Solid Edge part; units mm, degrees
sketch "Sketch1" plane through (0, 0, 0) normal (0, -1, 0) x (1, 0, 0)
  circle A0 centre (80.5127, 55.3877) radius 22.5
extrude "Protrusion1" add sketch "Sketch1" against normal blind 10
sketch "Sketch2" plane through (80.5127, 10, 55.3877) normal (0, 1, 0) x (0, 0, -1)
  circle A0 centre (0, 0) radius 2.95
extrude "ExtrudedCutout_5" cut sketch "Sketch2" against normal blind 4
sketch "Sketch3" plane through (80.5127, 6, 55.3877) normal (0, 1, 0) x (-1, 0, 0)
  circle A0 centre (0, 0) radius 1.05
extrude "Cutout1" cut sketch "Sketch3" against normal up to next
sketch "Sketch4" plane through (80.5127, 5, 51.1598) normal (0, -1, 0) x (1, 0, 0)
  circle A0 centre (0, 4.2279) radius 3.55
extrude "ExtrudedCutout_7" cut sketch "Sketch4" against normal blind 0.5
chamfer "Chamfer_2" distance 1.9 distance2 0.5 1 edges at (80.5127, 6, 58.3377) measured on face at (78.605, 6, 53.362)
sketch "Sketch5" plane through (80.5127, 10, 55.3877) normal (0, 1, 0) x (0, 0, 1)
  circle A0 centre (0, 0) radius 22.5
  circle A1 centre (0, 0) radius 3
extrude "ExtrudedProtrusion_4" add sketch "Sketch5" along normal blind 1.5
sketch "Sketch6" plane through (80.5127, 0, 55.3877) normal (0, -1, 0) x (0, 0, 1)
  line L0 (1.5, 9.61) -> (1.5, 5.61)
  arc A0 (5.61, 1.5) -> (1.5, 5.61) centre (1.5, 1.5) ccw
  line L1 (5.61, 1.5) -> (9.61, 1.5)
  arc A1 (9.61, 1.5) -> (9.61, -1.5) centre (9.61, 0) cw
  line L2 (9.61, -1.5) -> (5.61, -1.5)
  arc A2 (1.4978, -5.61) -> (5.61, -1.5) centre (1.4978, -1.4978) ccw
  line L3 (1.4978, -12.31) -> (1.4978, -5.61)
  arc A3 (-1.5, -12.31) -> (1.4978, -12.31) centre (-0.0011, -13.6341) ccw
  line L4 (-1.5, -5.61) -> (-1.5, -12.31)
  arc A4 (-5.61, -1.5) -> (-1.5, -5.61) centre (-1.5, -1.5) ccw
  line L5 (-9.61, -1.5) -> (-5.61, -1.5)
  arc A5 (-9.61, 1.5) -> (-9.61, -1.5) centre (-9.61, 0) ccw
  line L6 (-5.61, 1.5) -> (-9.61, 1.5)
  arc A6 (-5.61, 1.5) -> (-1.5, 5.61) centre (-1.5, 1.5) cw
  line L7 (-1.5, 9.61) -> (-1.5, 5.61)
  arc A7 (1.5, 9.61) -> (-1.5, 9.61) centre (0, 9.61) ccw
  dimension "D1" = 1.5
  dimension "D2" = 1.5
  dimension "D3" = 5.61
  dimension "D4" = 9.61
  dimension "D5" = 5.61
  dimension "D6" = 1.5
  dimension "D7" = 1.4978
  dimension "D8" = 9.61
extrude "ExtrudedCutout_9" cut sketch "Sketch6" against normal blind 6.7
sketch "Sketch7" plane through (80.5127, 11.5, 55.3877) normal (0, 1, 0) x (0, 0, -1)
  arc A0 (-7.5, 4.5) -> (-4.5, 7.5) centre (-7.9685, 7.9685) ccw
  line L0 (-3.5, 17.5) -> (-4.5, 7.5)
  arc A1 (-3.5, 17.5) -> (3.5, 17.5) centre (0, 17.15) cw
  line L1 (3.5, 17.5) -> (4.5, 7)
  arc A2 (4.5, 7) -> (7.5, 4.5) centre (7.8596, 7.9815) ccw
  line L2 (7.5, 4.5) -> (17.5, 3.5)
  arc A3 (17.5, 3.5) -> (17.5, -3.5) centre (17.15, 0) cw
  line L3 (7.5, -4.5) -> (17.5, -3.5)
  arc A4 (4.5, -7.5) -> (7.5, -4.5) centre (7.9657, -7.9657) cw
  line L4 (4.5, -7.5) -> (3.5, -17.5)
  arc A5 (-3.5, -17.5) -> (3.5, -17.5) centre (0, -17.15) ccw
  line L5 (-4.5, -7.5) -> (-3.5, -17.5)
  arc A6 (-7.5, -4.5) -> (-4.5, -7.5) centre (-7.9685, -7.9685) cw
  line L6 (-17.5, -3.5) -> (-7.5, -4.5)
  arc A7 (-17.5, 3.5) -> (-17.5, -3.5) centre (-17.15, 0) ccw
  line L7 (-7.5, 4.5) -> (-17.5, 3.5)
extrude "ExtrudedCutout_10" cut sketch "Sketch7" against normal blind 3.5
Input: part model. Units: mm. Frame: model coordinates. A direction names the side the tool comes from. Coordinates: 2 decimals unless noted, no trailing zeros. Loops run counter-clockwise (first coordinate to the right, second up) from the corner with the lowest first, then second, coordinate; pieces in that order, holes last. Notation, with made-up numbers: M 14,52 L 46,52 A16 ccw 46,59 Z; hole C 54.5,33 d11. An arc over 180 degrees is marked long. Use a Markdown table: item, result. Add a question column.
1) Section C-C, the plane x = 65.5. Return the cut outline in (y, z).
2) Set-up query: faces 1 (the cylindrical face through (101.18, 9.77, 55.46)), 2 (the cylindrical face through (84.887, 3.303, 50.95)), 3 (the flat face through (75.8, 0, 50.7)). Return all of +Z, -Z, +X, -X, +Y, -Y with unobstructed straight access to the full face (end or side cutting, diameter ignored); none if empty.
3) Pin query (flat end, axial travel): P1, Ø4.5, axis at x = 94.15, z = 55.39, coming from the +Y side; P2, Ø2, axis at x = 73, y = 4.5, coming from the +Z side; P3, Ø1.5, axis at x = 94, y = 9, coming from the -Z side. Return the tip coordinate at first contact, or that it passes through.
4) Section B-B, the plane z = 49. Return the cut outline in (x, y), plus the area to 3 significant figures.
5) Section A-A, the plane y = 9. Return the cut outline in (x, z).
6) Draft query along Z for faces 4 (the flat face through (71, 11.5, 60)), 5 (the cylindrical face through (80.44, 9.774, 76.054)), 6 (the flat face through (67.94, 9.77, 59.38)). Return one class per face: +Z half, -Z half, draft (parallel to the pull), parting line (faces both ways), or undercut.
7) Section D-D, the plane y = 5. Return the cut outline in (x, z), plus the area to 3 significant figures.
8) Line query: L1, parallel to Y at x = 84.5, z = 54.5; L2, parallel to X at y = 10.5, z = 48; L3, parallel to Z at x = 91.5, y = 9.25. Output: solid intervals per line, ascending. Write a range as from..to.
Answer below:
| question | item | result |
|---|---|---|
| 1 | outline | M 0,38.63 L 11.5,38.63 L 11.5,51.65 L 8,51.65 L 8,59.14 L 11.5,59.14 L 11.5,72.15 L 0,72.15 Z |
| 2 | face 1 | +Y |
| 2 | face 2 | -Y |
| 2 | face 3 | +Z, -Z, +X, -X, -Y |
| 3 | P1 | y = 8 |
| 3 | P2 | z = 76.92 |
| 3 | P3 | z = 36.84 |
| 4 | outline | M 58.94,0 L 79.01,0 L 79.01,6.7 L 82.01,6.7 L 82.01,0 L 102.09,0 L 102.09,11.5 L 85.36,11.5 L 85.36,8 L 75.71,8 L 75.71,11.5 L 58.94,11.5 Z |
| 4 | area | 442 mm2 |
| 5 | outline | C 80.51,55.39 d45; hole M 63.01,51.89 L 73.51,50.89 A3.5 cw 76.01,47.89 L 77.01,37.89 A3.52 ccw 84.01,37.89 L 85.01,47.89 A3.5 cw 88.01,50.89 L 98.01,51.89 A3.52 ccw 98.01,58.89 L 88.01,59.89 A3.5 cw 85.01,62.89 L 84.01,72.89 A3.52 ccw 77.01,72.89 L 76.01,62.89 A3.5 cw 73.01,59.89 L 63.01,58.89 A3.52 ccw Z |
| 6 | face 4 | draft |
| 6 | face 5 | undercut |
| 6 | face 6 | undercut |
| 7 | outline | C 80.51,55.39 d45; hole M 70.9,53.89 L 74.9,53.89 A4.11 ccw 79.01,49.78 L 79.01,45.78 A1.5 ccw 82.01,45.78 L 82.01,49.78 A4.11 ccw 86.12,53.89 L 92.82,53.89 A2 ccw long 92.82,56.89 L 86.12,56.89 A4.11 ccw 82.01,61 L 82.01,65 A1.5 ccw 79.01,65 L 79.01,61 A4.11 ccw 74.9,56.89 L 70.9,56.89 A1.5 ccw Z |
| 7 | area | 1,400 mm2 |
| 8 | L1 | 6.7..8 |
| 8 | L2 | 59.26..76, 85.03..101.77 |
| 8 | L3 | 35.75..51.24, 59.54..75.02 |
